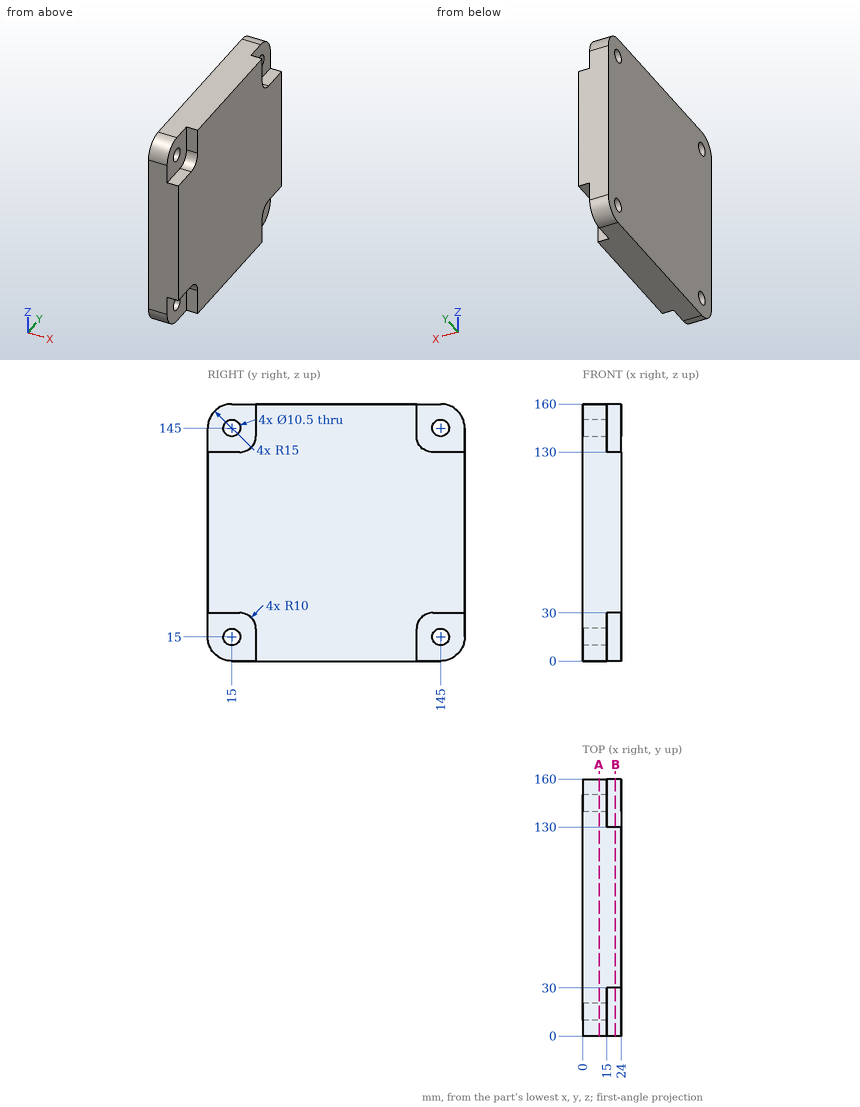
Geometry check sheet. Reference: drawing and pictorial views, mm from the part's lowest x, y, z. Give positions to 0.01 mm unless a question says otherwise; leave off trailing zeros. Order: outer loops, then holes, each group sorted by start corner. A loop starts at its lowest first (then second) coordinate and runs counter-clockwise, first axis right, second up. Notation, with made-up numbers: M -29.75,-2.5 L 18.25,-2.5 A17 ccw 18.25,13.5 Z; hole C -32.75,-8.5 d8. An arc over 180 degrees is marked long. Return JSON: item names as keys, results as strings. Group by question number.
1) Scan lines: line 1 (Z direction, x = 3.5, y = 145); line 2 (Y direction, x = 7.5, z = 148). Record each from-to range of solid material in increasing order.
2) Section check B-B on x = 20.25. Record the cut outline in (y, z), and give its area (3 significant figures).
3) Section check A-A on x = 10.25. Record the cut outline in (y, z), and give its area (3 significant figures).
4) Go/stop test with flat-tipped pins: pin 1 Ø12 at (y, z) = (15, 145) entering from +X; pin 2 Ø4.5 at (x, y) = (19, 14.5) entering from -Z; pin 3 Ø2.5 at (x, z) = (18, 6) entering from +Y. Record where each tip stops, or that it passes through.
Answer block:
{
 "1": {"line 1": "z = 0 to 9.75, 20.25 to 139.75, 150.25 to 160", "line 2": "y = 0.3 to 10.69, 19.31 to 140.69, 149.31 to 159.7"},
 "2": {"outline": "M 0,30 L 20,30 A10 cw 30,20 L 30,0 L 130,0 L 130,20 A10 cw 140,30 L 160,30 L 160,130 L 140,130 A10 cw 130,140 L 130,160 L 30,160 L 30,140 A10 cw 20,130 L 0,130 Z", "area": "22,100 mm^2"},
 "3": {"outline": "M 0,15 A15 ccw 15,0 L 145,0 A15 ccw 160,15 L 160,145 A15 ccw 145,160 L 15,160 A15 ccw 0,145 Z; hole C 15,15 d10.5; hole C 15,145 d10.5; hole C 145,15 d10.5; hole C 145,145 d10.5", "area": "25,100 mm^2"},
 "4": {"pin 1": "stops at x = 15", "pin 2": "stops at z = 30", "pin 3": "stops at y = 130"}
}
